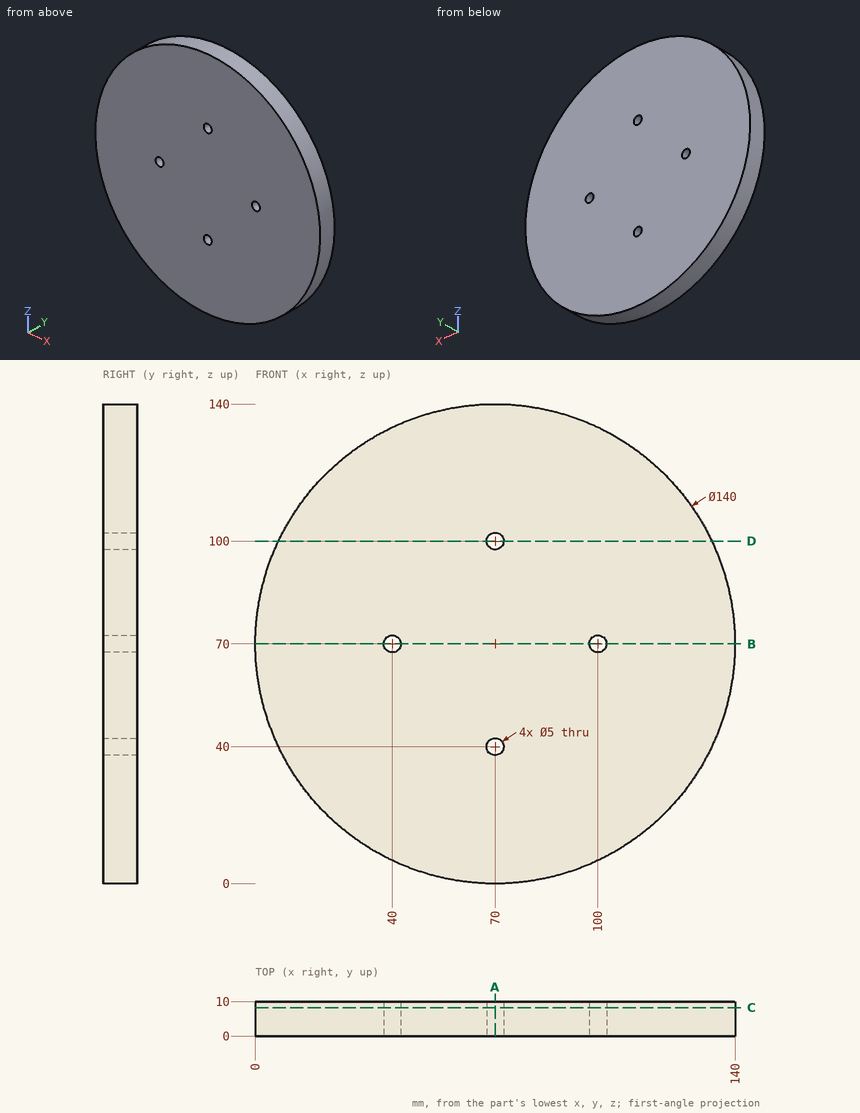
Check sheet for the drawn part. Datum: minimum x, y, z corner. Units: mm. Give positions to 0.01 mm unless a question says otherwise; leave off trailing zeros. Order: outer loops, then holes, each group sorted by start corner. A loop starts at its lowest first (then second) coordinate and runs counter-clockwise, first axis right, second up. Notation, with made-up numbers: (19, 37) -> (61, 37) arc R29 cw to (61, 57) -> close; hole circle Ø10 at (46.25, 1.5). An arc over 180 degrees is marked (long way). One line per item, written item: value.
(1) Sectioned sample at C-C on y = 8.25. Record the cut outline in (x, z).
Final values:
outline: circle Ø140 at (70, 70); hole circle Ø5 at (40, 70); hole circle Ø5 at (70, 40); hole circle Ø5 at (70, 100); hole circle Ø5 at (100, 70)
(2) Sectioned sample at D-D on z = 100. Record the cut outline in (x, y).
Final values:
outline: (6.75, 0) -> (67.5, 0) -> (67.5, 10) -> (6.75, 10) -> close; (72.5, 0) -> (133.25, 0) -> (133.25, 10) -> (72.5, 10) -> close
(3) Scan lines: line 1 along X through (y, z) = (7.75, 70); line 2 along X through (y, z) = (4.5, 69.5); line 3 along Z through (x, y) = (71, 2). Record each from-to range of solid material in increasing order. Write a range as [from, to].
Final values:
line 1: [0, 37.5], [42.5, 97.5], [102.5, 140]
line 2: [0, 37.55], [42.45, 97.55], [102.45, 140]
line 3: [0.01, 37.71], [42.29, 97.71], [102.29, 139.99]
(4) Sectioned sample at B-B on z = 70. Record the cut outline in (x, y), then the cut area to 3 significant figures.
Final values:
outline: (0, 0) -> (37.5, 0) -> (37.5, 10) -> (0, 10) -> close; (42.5, 0) -> (97.5, 0) -> (97.5, 10) -> (42.5, 10) -> close; (102.5, 0) -> (140, 0) -> (140, 10) -> (102.5, 10) -> close
area: 1,300 mm^2
(5) Gauge pin test, flat ends, axial feed: pin 1 (6 mm diameter, centred on y = 2, z = 89.5, fed in from -X); pin 2 (6 mm diameter, centred on x = 113.5, y = 7, fed in from -Z); pin 3 (4 mm diameter, centred on y = 7.5, z = 26, fed in from +X); pin 4 (4 mm diameter, centred on x = 100, z = 70, fed in from +Y). Record the tip position at first contact, or that the pin passes through.
Final values:
pin 1: x = 1.97
pin 2: z = 12.91
pin 3: x = 126
pin 4: through
(6) Sectioned sample at A-A on x = 70. Record the cut outline in (y, z), then the cut area to 3 significant figures.
Final values:
outline: (0, 0) -> (10, 0) -> (10, 37.5) -> (0, 37.5) -> close; (0, 42.5) -> (10, 42.5) -> (10, 97.5) -> (0, 97.5) -> close; (0, 102.5) -> (10, 102.5) -> (10, 140) -> (0, 140) -> close
area: 1,300 mm^2
